Here's how the part is built. I have some questions about the finished solid (model axes, mm). Face numbers are marked on the shaded views. A direction names the side the tool comes from. Round coordinates to 2 decimals unless told otherwise and drop trailing zeros. Loops run counter-clockwise (first coordinate to the right, second up) from the corner with the lowest first, then second, coordinate; pieces in that order, holes last. Notation, with made-up numbers: M 80.5,69 L 90.5,69 A34 cw 90.5,106 Z; hole C 70,58 d5. An arc over 180 degrees is marked long. Answer as a JSON object with one key per item and string values.
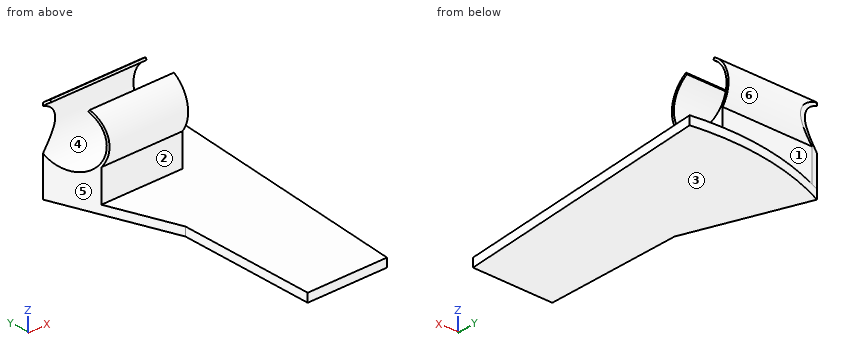
from build123d import *

# Parameters (mm, degrees)
F1_DEPTH = 3.81
F2_W     = 54.356
F2_H     = 38.1
F3_DEPTH = 50.8
F5_DEPTH = 54.357
F7_DEPTH = 38.6182152336


with BuildPart() as f1:
    # F0 (on Top) → F1 (new body)
    with BuildSketch(Plane.XY):
        with BuildLine():
            ThreePointArc((32.3535154368, 26.1046796118), (-0.7575616132, 26.3503201986), (-32.5620487044, 17.1373747646))
            Line((-32.5620487044, 17.1373747646), (32.3535154368, 26.1046796118))
        make_face()
        Polygon((32.3535154368, 26.1046796118), (-32.5620487044, 17.1373747646), (-14.3325939581, -32.94764052), (-14.3325939581, -93.2497044648), (21.0546860419, -93.2497044648), align=None)
    extrude(amount=F1_DEPTH)

    # F2 (on face) → F3 (join)
    with BuildSketch(Plane.XY.offset(3.81)):
        with Locations((-16.1494093879, 7.7088556692)):
            Rectangle(F2_W, F2_H)
        with BuildLine():
            Line((11.0285906121, 26.7588556692), (2.554207671, 26.7588556692))
            ThreePointArc((2.554207671, 26.7588556692), (-15.3877109544, 23.3488645961), (-32.5620487044, 17.1373747646))
            Line((-32.5620487044, 17.1373747646), (-22.1967154377, -11.3411443308))
            Line((-22.1967154377, -11.3411443308), (11.0285906121, -11.3411443308))
            Line((11.0285906121, -11.3411443308), (11.0285906121, 26.7588556692))
        make_face()
    extrude(amount=F3_DEPTH)

    # F4 (on face) → F5 (cut, through all)
    with BuildSketch(Plane.YZ.offset(11.0285906121)):
        with BuildLine():
            Line((0.7238556692, 38.6172152336), (1.2088556692, 37.777170592))
            ThreePointArc((1.2088556692, 37.777170592), (7.7088556692, 13.5188403428), (14.2088556692, 37.777170592))
            Line((14.2088556692, 37.777170592), (14.6938556692, 38.6172152336))
            ThreePointArc((14.6938556692, 38.6172152336), (21.4068223617, 29.2623068525), (18.8143789297, 18.0436852935))
            Line((18.8143789297, 18.0436852935), (18.8143789297, 3.81))
            Line((18.8143789297, 3.81), (26.7588556692, 3.81))
            Line((26.7588556692, 3.81), (26.7588556692, 54.61))
            Line((26.7588556692, 54.61), (-11.3411443308, 54.61))
            Line((-11.3411443308, 54.61), (-11.3411443308, 3.81))
            Line((-11.3411443308, 3.81), (-3.3966675913, 3.81))
            Line((-3.3966675913, 3.81), (-3.3966675913, 18.0436852935))
            ThreePointArc((-3.3966675913, 18.0436852935), (-5.9891110233, 29.2623068525), (0.7238556692, 38.6172152336))
        make_face()
    extrude(amount=-F5_DEPTH, mode=Mode.SUBTRACT)

    # F6 (on face) → F7 (cut, through all)
    with BuildSketch(Plane(origin=(0, 0, 0), x_dir=(1, 0, 0), z_dir=(0, 0, -1))):
        with BuildLine():
            ThreePointArc((-11.1417521231, -24.4255824736), (-22.048556528, -21.3594577958), (-32.5620487044, -17.1373747646))
            Line((-32.5620487044, -17.1373747646), (-22.9622920053, 9.2377399985))
            Line((-22.9622920053, 9.2377399985), (-52.2691048682, 17.8252514452))
            Line((-52.2691048682, 17.8252514452), (-60.0504353642, -34.5690436661))
            Line((-60.0504353642, -34.5690436661), (-11.1417521231, -24.4255824736))
        make_face()
    extrude(amount=-F7_DEPTH, mode=Mode.SUBTRACT)


solid = f1.part
Item 1: I want a section at D-D, the plane y = 4. Please give me the cut outline in (x, z).
Resolved:
{"outline": "M -27.78,0 L 30.26,0 L 30.26,3.81 L 11.03,3.81 L 11.03,14.06 L -27.78,14.06 Z"}
Item 2: I'm going to push flat-ended pins straight in: pin 1 Ø15.5 at (x, z) = (-6, 12.5) entering from -Y; pin 2 Ø1.5 at (x, y) = (-14, -50) entering from +Z; pin 3 Ø15.5 at (x, z) = (-4, 9.5) entering from +Y. Where does each tip first touch, or does it pass through?
Resolved:
{"pin 1": "y = -4.78", "pin 2": "z = 3.81", "pin 3": "y = 26.61"}
Item 3: I want a section at A-A, the plane z = 31. Please give me the cut outline in (x, y).
Resolved:
{"outline": "M -26.04,19.91 L 11.03,19.91 L 11.03,20.94 L -23.26,20.94 A105.12 ccw Z; M -24.69,-4.49 L -24.31,-5.52 L 11.03,-5.52 L 11.03,-4.49 Z"}
Item 4: I want a section at C-C, the plane z = 26. Please give me the cut outline in (x, y).
Resolved:
{"outline": "M -24.4,-5.28 L -24.05,-6.25 L 11.03,-6.25 L 11.03,-5.28 Z; M -23.93,20.7 L 11.03,20.7 L 11.03,21.67 L -21.12,21.67 A105.12 ccw Z"}
Item 5: Please list where these lines run through material, in increasing order: probe 1 along Z at (x, y) = (11, -84); probe 2 along Y at (x, z) = (-14.5, 28.5); probe 3 along Y at (x, z) = (-4, 6.5). Write a range as from..to.
Resolved:
{"probe 1": "0..3.81", "probe 2": "-6.12..-5.14, 20.56..21.54", "probe 3": "-3.4..18.81"}
Item 6: If we mould it in two halves opening along Z, with no side actions, what happens to the marked faces 3, 4, 5 and 6? For each: pulls with the +Z half, pulls with the -Z half, needs draft (parallel to the pull), parting line crosses it, or undercut.
Resolved:
{"face 3": "pulls with the -Z half", "face 4": "undercut", "face 5": "needs draft", "face 6": "undercut"}
Item 7: On a 3-axis mill with a long thin cutter (end or side, diameter ignored), from which of +Z, -Z, +X, -X, +Y, -Y can I reach the whole of each face in a straight line? I mean the marked faces 1 and 2. Say none if no direction works.
Resolved:
{"face 1": "+X, -X, +Y", "face 2": "+X, -X, -Y"}
Item 8: I want a section at B-B, the plane x = -19. Please give me the cut outline in (y, z).
Resolved:
{"outline": "M -20.12,0 L 22.3,0 L 22.3,3.81 L 18.81,3.81 L 18.81,18.04 A13.97 ccw 14.69,38.62 L 14.21,37.78 A13 cw long 1.21,37.78 L 0.72,38.62 A13.97 ccw -3.4,18.04 L -3.4,3.81 L -20.12,3.81 Z"}
